```python
from build123d import *

# Parameters (mm, degrees)
SKETCH1_W           = 15
SKETCH1_H           = 8
SKETCH1_R           = 1.6
BOSS_EXTRUDE1_DEPTH = 2
SKETCH2_R           = 1.125
CUT_EXTRUDE1_DEPTH  = 28.572631358
FILLET2_R           = 10
FILLET3_R           = 2
FILLET6_R           = 2
FILLET5_R           = 0.5


with BuildPart() as part:
    # Sketch1 → Boss-Extrude1 (new, symmetric)
    with BuildSketch(Plane.XY):
        Polygon((-16.5, -9), (16.5, -9), (16.5, 9), (3, 9), (3, 31), (-3, 31), (-3, 9), (-16.5, 9), align=None)
        Rectangle(SKETCH1_W, SKETCH1_H, mode=Mode.SUBTRACT)
        with Locations((0, 27.95)):
            Circle(SKETCH1_R, mode=Mode.SUBTRACT)
    extrude(amount=BOSS_EXTRUDE1_DEPTH, both=True)

    # Sketch2 → Cut-Extrude1 (cut, through all)
    with BuildSketch(Plane(origin=(0, 9, 0), x_dir=(1, 0, 0), z_dir=(0, 1, 0))):
        with Locations(Location((-14.5, 0, 0), (0, 0, 180))):
            Circle(SKETCH2_R)
        with Locations(Location((14.5, 0, 0), (0, 0, 180))):
            Circle(SKETCH2_R)
    extrude(amount=-CUT_EXTRUDE1_DEPTH, mode=Mode.SUBTRACT)

    # Fillet2
    fillet2_edges = [part.edges().sort_by_distance(p)[0] for p in [
        (-3, 9, 0),
        (3, 9, 0),
    ]]
    fillet(fillet2_edges, radius=FILLET2_R)

    # Fillet3
    fillet3_edges = [part.edges().sort_by_distance(p)[0] for p in [
        (-3, 31, 0),
        (3, 31, 0),
    ]]
    fillet(fillet3_edges, radius=FILLET3_R)

    # Fillet6
    fillet6_edges = [part.edges().sort_by_distance(p)[0] for p in [
        (-7.5, 4, 0),
        (-7.5, -4, 0),
        (7.5, -4, 0),
        (7.5, 4, 0),
    ]]
    fillet(fillet6_edges, radius=FILLET6_R)

    # Fillet5
    fillet5_edges = [part.edges().sort_by_distance(p)[0] for p in [
        (16.5, 0, -2),
        (-16.5, 0, -2),
        (16.5, 9, 0),
        (16.5, -9, 0),
        (-16.5, -9, 0),
        (-16.5, 9, 0),
        (16.5, 0, 2),
        (14.75, 9, 2),
        (-14.75, 9, -2),
        (-14.75, 9, 2),
        (3, 24, -2),
        (3, 24, 2),
        (-5.928932188, 11.928932188, -2),
        (-5.928932188, 11.928932188, 2),
        (5.928932188, 11.928932188, -2),
        (5.928932188, 11.928932188, 2),
        (0, 31, -2),
        (0, 31, 2),
        (-3, 24, -2),
        (-2.414213562, 30.414213562, -2),
        (2.414213562, 30.414213562, -2),
        (-3, 24, 2),
        (-2.414213562, 30.414213562, 2),
        (2.414213562, 30.414213562, 2),
        (-16.5, 0, 2),
        (14.75, 9, -2),
    ]]
    fillet(fillet5_edges, radius=FILLET5_R)


solid = part.part
```
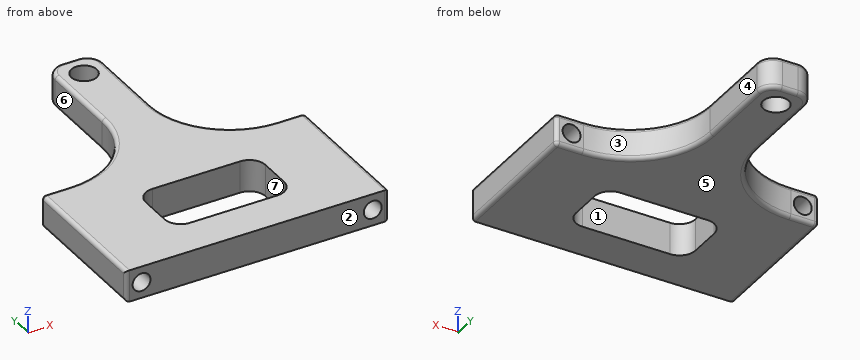
Here's how the part is built. I have some questions about the finished solid (model axes, mm). Face numbers are marked on the shaded views. A direction names the side the tool comes from. Round coordinates to 2 decimals unless told otherwise and drop trailing zeros. Write each loop counter-clockwise with the first axis right and the second up, starting at its lowest first coordinate (ties: lowest second). Pieces come first, ordered by that corner, then holes. Notation, with made-up numbers: M 86.25,-18 L 117.25,-18 A21 ccw 117.25,-2 Z; hole C -5,84 d7. An arc over 180 degrees is marked long. Answer as CSV lines item,"result". Start each with the question number.
1. I'm going to push flat-ended pins straight in: pin 1 Ø1.5 at (x, z) = (-11, -1.5) entering from +Y; pin 2 Ø8 at (x, y) = (3, -2) entering from -Z; pin 3 Ø2 at (x, z) = (2.5, 0.5) entering from +Y; pin 4 Ø1.3 at (x, z) = (-14.5, 0) entering from +Y. Where does each tip first touch, or does it pass through?
2. Suppose I cut it at B-B on z = 0. Count the separate pieces of the cut face and the enclosed holes in it, then the cut area to 3 significant figures.
3. Suppose I cut it at C-C on y = 27.95. Write out the boundary of the cut face in (x, z), then the cut area to 3 significant figures.
4. Thinking about a two-plate mould opening in Y: for the marked faces 1, 2 and 3, which applies, released by +Y, released by -Y, zero draft, split by the parting line, or undercut?
5. I need wall thicknesses on probe 1 along Y at (x, z) = (0, -0.65); probe 2 along Z at (x, y) = (-14.5, -3) (3 decimals); probe 3 along X at (y, z) = (0, -0.95). Which ranges of each line are inside material? Lowest first, please.
6. Suppose I cut it at D-D on y = 0.5. Write out the boundary of the cut face in (x, z) (3 decimals), then the cut area to 3 significant figures.
7. Suppose I cut it at A-A on x = 0. Write out the boundary of the cut face in (y, z).
8. On a 3-axis mill with a long thin cutter (end or side, diameter ignored), from which of +Z, -Z, +X, -X, +Y, -Y can I reach the whole of each face in a straight line? I mean the marked faces 4, 5, 6 and 7. Say none if no direction works.
Check result:
1,pin 1,"stops at y = 9.39"
1,pin 2,"stops at z = -2"
1,pin 3,"stops at y = 30.94"
1,pin 4,"passes through"
2,separate pieces,"3"
2,enclosed holes,"2"
2,area,"561 mm2"
3,outline,"M -3,-1.5 A0.5 ccw -2.5,-2 L -1.6,-2 L -1.6,2 L -2.5,2 A0.5 ccw -3,1.5 Z; M 1.6,-2 L 2.5,-2 A0.5 ccw 3,-1.5 L 3,1.5 A0.5 ccw 2.5,2 L 1.6,2 Z"
3,area,"11.0 mm2"
4,face 1,"undercut"
4,face 2,"released by -Y"
4,face 3,"released by +Y"
5,probe 1,"y = -9 to -4, 4 to 26.35, 29.55 to 31"
5,probe 2,"z = -2 to -1.125, 1.125 to 2"
5,probe 3,"x = -16.5 to -15.1, -13.9 to -7.5, 7.5 to 13.9, 15.1 to 16.5"
6,outline,"M -16.5,-1.5 A0.5 ccw -16,-2 L -7.5,-2 L -7.5,2 L -16,2 A0.5 ccw -16.5,1.5 Z; M 7.5,-2 L 16,-2 A0.5 ccw 16.5,-1.5 L 16.5,1.5 A0.5 ccw 16,2 L 7.5,2 Z; hole C -14.5,0 d2.25; hole C 14.5,0 d2.25"
6,area,"63.8 mm2"
7,outline,"M -9,-2 L -4,-2 L -4,2 L -9,2 Z; M 4,-2 L 26.35,-2 L 26.35,2 L 4,2 Z; M 29.55,-2 L 30.5,-2 A0.5 ccw 31,-1.5 L 31,1.5 A0.5 ccw 30.5,2 L 29.55,2 Z"
8,face 4,"+Z, -Z, +X, +Y"
8,face 5,"-Z, +X, -X, +Y, -Y"
8,face 6,"+Z, -Z, -X, +Y"
8,face 7,"+Z, -Z"
